Input: part model. Units: mm. Frame: model coordinates. A direction names the side the tool comes from. Coordinates: 2 decimals unless noted, no trailing zeros. Order: outer loops, then holes, each group sorted by start corner. A loop starts at its lowest first (then second) coordinate and runs counter-clockwise, first axis right, second up. Notation, with made-up numbers: M 78,55 L 90,55 A12 ccw 90,66 Z; hole C -0.5,72 d7. An arc over 180 degrees is marked long. One line per item, written item: value.
```python
from build123d import *

# Parameters (mm, degrees)
CROQUIS1_W                          = 19.75
CROQUIS1_H                          = 35
SALIENTE_EXTRUIR1_DEPTH             = 2.5
CROQUIS2_W                          = 3
CROQUIS2_H                          = 9.5
CORTAR_EXTRUIR1_DEPTH               = 21.24884256
CROQUIS3_W                          = 29.75
CROQUIS3_H                          = 15.75
SALIENTE_EXTRUIR2_DEPTH             = 2.5
CROQUIS7_R                          = 6.25
SALIENTE_EXTRUIR4_DEPTH             = 12
SALIENTE_EXTRUIR4_DIRECTION_2_REACH = 25.103
CROQUIS4_R                          = 2.5
SALIENTE_EXTRUIR3_DEPTH             = 15
CROQUIS5_R                          = 1.25
CORTAR_EXTRUIR2_DEPTH               = 41.688796062
CROQUIS10_R                         = 4.125
CORTAR_EXTRUIR3_DEPTH               = 12
CHAFL_N1_SIZE                       = 1
REDONDEO1_R                         = 2
CHAFL_N2_SIZE                       = 2.75
REDONDEO2_R                         = 5
SALIENTE_EXTRUIR5_DEPTH             = 2.5


with BuildPart() as part:
    # Croquis1 → Saliente-Extruir1 (new body)
    with BuildSketch(Plane.XY):
        Rectangle(CROQUIS1_W, CROQUIS1_H)
    extrude(amount=SALIENTE_EXTRUIR1_DEPTH)

    # Croquis2 → Cortar-Extruir1 (cut, through all)
    with BuildSketch(Plane.XY.offset(2.5)):
        with Locations((0, -12.75)):
            Rectangle(CROQUIS2_W, CROQUIS2_H)
    extrude(amount=-CORTAR_EXTRUIR1_DEPTH, mode=Mode.SUBTRACT)

    # Croquis3 → Saliente-Extruir2 (add, through all)
    with BuildSketch(Plane.XY.offset(2.5)):
        with Locations((0, 9.625)):
            Rectangle(CROQUIS3_W, CROQUIS3_H)
    extrude(amount=-SALIENTE_EXTRUIR2_DEPTH)

    # Croquis7 → Saliente-Extruir4 (add)
    with BuildSketch(Plane.XY.offset(2.5)):
        with Locations((0, 17.5)):
            Circle(CROQUIS7_R)
    extrude(amount=SALIENTE_EXTRUIR4_DEPTH)

    # Saliente-Extruir4 direction 2: up to this face of the body (flat: up to its plane)
    saliente_extruir4_direction_2_end = Plane(part.part.faces().sort_by_distance((0, 2.291145992, 0))[0])
    # Croquis7 → Saliente-Extruir4 direction 2 (add, up to the picked face)
    with BuildSketch(Plane.XY.offset(2.5), mode=Mode.PRIVATE) as saliente_extruir4_direction_2_sk1:
        with Locations((0, 17.5)):
            Circle(CROQUIS7_R)
    saliente_extruir4_direction_2_tool1 = split(extrude(saliente_extruir4_direction_2_sk1.sketch, amount=-SALIENTE_EXTRUIR4_DIRECTION_2_REACH, mode=Mode.PRIVATE), bisect_by=saliente_extruir4_direction_2_end, keep=Keep.BOTH, mode=Mode.PRIVATE)
    add(saliente_extruir4_direction_2_tool1.solids().sort_by(Axis((0, 17.5, 2.5), (0, 0, -1)))[0])

    # Croquis4 → Saliente-Extruir3 (add)
    with BuildSketch(Plane.XY.offset(14.5)):
        with Locations((0, 17.5)):
            Circle(CROQUIS4_R)
    extrude(amount=SALIENTE_EXTRUIR3_DEPTH)

    # Croquis5 → Cortar-Extruir2 (cut, through all)
    with BuildSketch(Plane.XY.offset(29.5)):
        with Locations((0, 17.5)):
            Circle(CROQUIS5_R)
    extrude(amount=-CORTAR_EXTRUIR2_DEPTH, mode=Mode.SUBTRACT)

    # Croquis10 → Cortar-Extruir3 (cut)
    with BuildSketch(Plane(origin=(0, 0, 0), x_dir=(-1, 0, 0), z_dir=(0, 0, -1))):
        with Locations((0, 17.5)):
            Circle(CROQUIS10_R)
    extrude(amount=-CORTAR_EXTRUIR3_DEPTH, mode=Mode.SUBTRACT)

    # Chaflán1
    chafl_n1_edges = [part.edges().sort_by_distance(p)[0] for p in [
        (-2.5, 17.5, 29.5),
        (4.125, 17.5, 0),
    ]]
    chamfer(chafl_n1_edges, length=CHAFL_N1_SIZE)

    # Redondeo1
    redondeo1_edges = [part.edges().sort_by_distance(p)[0] for p in [
        (1.5, -17.5, 1.25),
        (-1.5, -17.5, 1.25),
        (-14.875, 17.5, 1.25),
        (14.875, 1.75, 1.25),
        (-14.875, 1.75, 1.25),
        (14.875, 17.5, 1.25),
        (9.875, -17.5, 1.25),
        (-9.875, -17.5, 1.25),
    ]]
    fillet(redondeo1_edges, radius=REDONDEO1_R)

    # Chaflán2
    chafl_n2_edges = [part.edges().sort_by_distance(p)[0] for p in [
        (-6.25, 17.5, 14.5),
        (4.125, 17.5, 12),
    ]]
    chamfer(chafl_n2_edges, length=CHAFL_N2_SIZE)

    # Redondeo2
    # the kernel refuses this fillet: 5 mm, written as the material it adds along each edge
    with BuildSketch(Plane(origin=(0, 17.5, 14.5), x_dir=(1, 0, 0), z_dir=(0, -1, 0))) as redondeo2_piece_1:
        with BuildLine():
            CenterArc((7.5, 3), REDONDEO2_R, 180, 36.869897646)
            Line((2.5, 3), (2.4, 3))
            Line((2.4, 3), (2.4, 0))
            Line((2.4, 0), (2.5, -0.1))
            ThreePointArc((2.5, -0.1), (3, -0.1), (3.42, -0.06))
            Line((3.42, -0.06), (3.5, 0))
        make_face()
    revolve(axis=Axis((0, 17.5, 14.5), (0, 0, 1)))

    # Croquis11 → Saliente-Extruir5 (add)
    with BuildSketch(Plane(origin=(0, 0, 0), x_dir=(-1, 0, 0), z_dir=(0, 0, -1))):
        with BuildLine():
            ThreePointArc((-6.25, 17.5), (-4.419417386, 21.919417379), (-1e-08, 23.75))
            Line((-1e-08, 23.75), (-12.875, 23.75))
            ThreePointArc((-12.875, 23.75), (-14.289213562, 23.164213562), (-14.875, 21.75))
            Line((-14.875, 21.75), (-14.875, 15.5))
            ThreePointArc((-14.875, 15.5), (-14.289213562, 16.914213562), (-12.875, 17.5))
            Line((-12.875, 17.5), (-6.25, 17.5))
        make_face()
        with BuildLine():
            ThreePointArc((-1e-08, 23.75), (4.419417379, 21.919417386), (6.25, 17.5))
            Line((6.25, 17.5), (12.875, 17.5))
            ThreePointArc((12.875, 17.5), (14.289213562, 16.914213562), (14.875, 15.5))
            Line((14.875, 15.5), (14.875, 21.75))
            ThreePointArc((14.875, 21.75), (14.289213562, 23.164213562), (12.875, 23.75))
            Line((12.875, 23.75), (-1e-08, 23.75))
        make_face()
    extrude(amount=-SALIENTE_EXTRUIR5_DEPTH)


solid = part.part
```
(1) First-contact query: pin 1 (1 mm diameter, centred on x = 5.5, y = 18, fed in from +Z); pin 2 (2 mm diameter, centred on x = 10.5, z = 1, fed in from -Y); pin 3 (2 mm diameter, centred on y = -11, z = 2, fed in from -X) (3 decimals); pin 4 (2 mm diameter, centred on x = 0, y = 17.5, fed in from -Z). Flat tips, straight axial feed; report the tip coordinate or a pass-through.
Data:
pin 1: stops at z = 12.98
pin 2: stops at y = -16.67
pin 3: stops at x = -9.875
pin 4: passes through
(2) Access query for faces 1 (the flat face through (-11, 1.75, 1)), 2 (the cylindrical face through (2.1, -16.93, 1.23)), 3 (the flat face through (-14.875, 13, 1)). Directions: +Z, -Z, +X, -X, +Y, -Y. A direction counts if a zero-diameter tool reaches every point of the face in a straight line with its end or side. Return the directions, or none.
Data:
face 1: +Z, -Z, -X, -Y
face 2: +Z, -Z, -Y
face 3: +Z, -Z, -X, +Y, -Y
(3) Cut plane B-B on y = -10. Output: boundary loops of the cut face in (x, z) (3 decimals), plus the area to 3 significant figures.
Data:
outline: M -9.875,0 L -1.5,0 L -1.5,2.5 L -9.875,2.5 Z; M 1.5,0 L 9.875,0 L 9.875,2.5 L 1.5,2.5 Z
area: 41.9 mm2
(4) Cut plane D-D on z = 14. Output: boundary loops of the cut face in (x, y), plus the area to 3 significant figures.
Data:
outline: C 0,17.5 d8; hole C 0,17.5 d2.5
area: 45.4 mm2
(5) Draft query along X for faces 4 (the cylindrical face through (-14.305, 2.351, 1.232)), 5 (the cylindrical face through (9.305, -16.899, 1.268)), 6 (the cylindrical face through (0.54, 21.59, 5.07)). Return one class per face: released by +X, released by -X, zero draft, split by the parting line, or undercut.
Data:
face 4: released by -X
face 5: released by +X
face 6: undercut
(6) Cut plane A-A on y = 17.5. Output: boundary loops of the cut face in (x, z) (3 decimals).
Data:
outline: M -14.875,0 L -5.125,0 L -4.125,1 L -4.125,9.25 L -1.375,12 L -1.25,12 L -1.25,29.5 L -1.5,29.5 L -2.5,28.5 L -2.5,17.5 A5 cw -3.5,14.5 L -6.25,11.75 L -6.25,2.5 L -14.875,2.5 Z; M 1.25,12 L 1.375,12 L 4.125,9.25 L 4.125,1 L 5.125,0 L 14.875,0 L 14.875,2.5 L 6.25,2.5 L 6.25,11.75 L 3.5,14.5 A5 cw 2.5,17.5 L 2.5,28.5 L 1.5,29.5 L 1.25,29.5 Z
(7) Ray query, line 1 (Y direction, x = 0, z = 25.25); line 2 (Z direction, x = 2.5, y = 1.5); line 3 (X direction, y = 16.5, z = 19). Return the intervals inside material, ascending. Write a range as from..to.
Data:
line 1: y = 15..16.25, 18.75..20
line 2: z = 0..2.5
line 3: x = -2.29..-0.75, 0.75..2.29
(8) Cut plane C-C on x = 11.25. Output: boundary loops of the cut face in (y, z).
Data:
outline: M 1.75,0 L 23.75,0 L 23.75,2.5 L 1.75,2.5 Z
